Check sheet for the modelled part. Datum: model origin and axes. Units: mm. Face numbers are marked on the shaded views. A direction names the side the tool comes from. Coordinates: 2 decimals unless noted, no trailing zeros. Loops run counter-clockwise (first coordinate to the right, second up) from the corner with the lowest first, then second, coordinate; pieces in that order, holes last.
```python
from build123d import *

# Parameters (mm, degrees)
F0_R     = 5.1562
F0_R_2   = 6.858
F1_DEPTH = 12.7
F2_R     = 5.1562
F2_R_2   = 6.858
F3_DEPTH = 12.7
F4_R     = 6.0071
F5_DEPTH = 12.7
F6_R     = 6.0071
F7_DEPTH = 12.7


with BuildPart() as f1:
    # F0 (on Front) → F1 (new body, symmetric)
    with BuildSketch(Plane.XZ):
        Circle(F0_R)
        Circle(F0_R_2)
        Circle(F0_R, mode=Mode.SUBTRACT)
    extrude(amount=F1_DEPTH, both=True)

    # F2 (on Right) → F3 (join, symmetric)
    with BuildSketch(Plane.YZ):
        Circle(F2_R)
        Circle(F2_R_2)
        Circle(F2_R, mode=Mode.SUBTRACT)
    extrude(amount=F3_DEPTH, both=True)

    # F4 (on Right) → F5 (cut, symmetric)
    with BuildSketch(Plane.YZ):
        Circle(F4_R)
    extrude(amount=F5_DEPTH, both=True, mode=Mode.SUBTRACT)

    # F6 (on Front) → F7 (cut, symmetric)
    with BuildSketch(Plane.XZ):
        Circle(F6_R)
    extrude(amount=F7_DEPTH, both=True, mode=Mode.SUBTRACT)


solid = f1.part
```
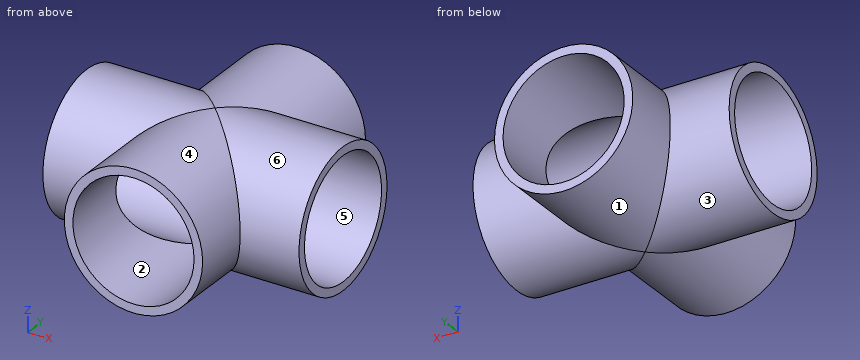
1) Section check D-D on y = -7.5. Enter the section's corners in (x, z), plus the area to 3 significant figures.
Answer sheet:
outline: circle Ø13.72 at (0, 0); hole circle Ø12.01 at (0, 0)
area: 34.4 mm2
2) Scan lines: line 1 (Z direction, x = 0, y = 5.5); line 2 (Y direction, x = -10.75, z = 4.5). Record each from-to range of solid material in increasing order.
Answer sheet:
line 1: z = -6.86 to -6.01, 6.01 to 6.86
line 2: y = -5.18 to -3.98, 3.98 to 5.18
3) Section check C-C on y = 3.75. Enter the section's corners in (x, z), plus the area to 3 significant figures.
Answer sheet:
outline: (-12.7, -5.74) - (-3.75, -5.74) arc R6.86 ccw to (3.75, -5.74) - (12.7, -5.74) - (12.7, -4.69) - (3.75, -4.69) arc R6.01 cw to (-3.75, -4.69) - (-12.7, -4.69) - close; (-12.7, 4.69) - (-3.75, 4.69) arc R6.01 cw to (3.75, 4.69) - (12.7, 4.69) - (12.7, 5.74) - (3.75, 5.74) arc R6.86 ccw to (-3.75, 5.74) - (-12.7, 5.74) - close
area: 51.2 mm2
4) Set-up check for the marked faces 3, 4, 5 and 6: record each of +Z, -Z, +X, -X, +Y, -Y from which the full face is reachable in a straight line by a thin tool's end or side.
Answer sheet:
face 3: -X
face 4: -Y
face 5: +X, -X
face 6: +X
5) Section check B-B on x = -5.5. Enter the section's corners in (y, z), plus the area to 3 significant figures.
Answer sheet:
outline: (-12.7, -4.1) - (-5.5, -4.1) arc R6.86 ccw to (5.5, -4.1) - (12.7, -4.1) - (12.7, -2.42) - (5.5, -2.42) arc R6.01 cw to (-5.5, -2.42) - (-12.7, -2.42) - close; (-12.7, 2.42) - (-5.5, 2.42) arc R6.01 cw to (5.5, 2.42) - (12.7, 2.42) - (12.7, 4.1) - (5.5, 4.1) arc R6.86 ccw to (-5.5, 4.1) - (-12.7, 4.1) - close
area: 70.9 mm2
6) Depth check by flat-ended pin: pin 1 (3 mm diameter, centred on y = 9.5, z = -2.5, fed in from +X); pin 2 (10 mm diameter, centred on x = 4, y = 5.5, fed in from +Z); pin 3 (6 mm diameter, centred on x = 10, z = 0.5, fed in from +Y); pin 4 (2 mm diameter, centred on y = 9, z = 0.5, fed in from -X). Enter the tip coordinate at first touch or a pass-through.
Answer sheet:
pin 1: stops at x = 6.78
pin 2: stops at z = 6.86
pin 3: stops at y = 6.86
pin 4: stops at x = -6.86
7) Section check A-A on z = 0. Enter the section's corners in (x, y), plus the area to 3 significant figures.
Answer sheet:
outline: (-12.7, -6.86) - (-6.86, -6.86) - (-6.86, -12.7) - (-6.01, -12.7) - (-6.01, -6.01) - (-12.7, -6.01) - close; (-12.7, 6.01) - (-6.01, 6.01) - (-6.01, 12.7) - (-6.86, 12.7) - (-6.86, 6.86) - (-12.7, 6.86) - close; (6.01, -12.7) - (6.86, -12.7) - (6.86, -6.86) - (12.7, -6.86) - (12.7, -6.01) - (6.01, -6.01) - close; (6.01, 6.01) - (12.7, 6.01) - (12.7, 6.86) - (6.86, 6.86) - (6.86, 12.7) - (6.01, 12.7) - close
area: 42.7 mm2
8) Mould release check, pull along X, two halves, no side actions. Record for the marked faces 1 and 2: +X half, -X half, draft (parallel to the pull), parting line (faces both ways), or undercut.
Answer sheet:
face 1: parting line
face 2: undercut
